```python
from build123d import *

# Parameters (mm, degrees)
F1_DEPTH = 100
F3_DEPTH = 100


with BuildPart() as f1:
    # F0 (on Front) → F1 (new body, symmetric)
    with BuildSketch(Plane.XZ):
        Polygon((450, -325), (450, 325), (150, 325), (150, 75), (-150, 75), (-150, 325), (-450, 325), (-450, -325), align=None)
    extrude(amount=F1_DEPTH, both=True)

    # F2 (on face) → F3 (join, symmetric)
    with BuildSketch(Plane.XZ.offset(100)):
        Polygon((-450, 325), (-450, -325), (-150, -325), align=None)
        Polygon((450, 325), (150, -325), (450, -325), align=None)
    extrude(amount=F3_DEPTH, both=True)


solid = f1.part
```
Could you check a few things on this model? Use its own coordinates, in mm. A direction names the side the tool comes from. Give positions to 0.01 mm unless a question says otherwise; leave off trailing zeros. Order: outer loops, then holes, each group sorted by start corner. A loop starts at its lowest first (then second) coordinate and runs counter-clockwise, first axis right, second up.
Q1. If I drill on line 1 along X through (y, z) = (28, 139); line 2 along Y through (x, z) = (222, 250.5); line 3 along Z through (x, y) = (-42.5, -1.5), over which ranges is the centre line in solid material (lowest first)?
Q2. Suppose I cut it at B-B, the plane z = 149. Write out the boundary of the cut face in (x, y).
Q3. I'm going to push a flat-ended pin straight in: P1, Ø10, axis at x = -122, z = -181.5, coming from the -Y side. Where does the tip first touch, or does it pass through?
Q4. Suppose I cut it at C-C, the plane y = -23.5. Write out the boundary of the cut face in (x, z), and give its area (3 significant figures).
Q5. Suppose I cut it at D-D, the plane z = -255. Write out the boundary of the cut face in (x, y).
Q6. We'd pull the mould along X, two halves only. Please class faces 4 (the flat face through (450, -52, -5)), 5 (the flat face through (-6, -52, -325)), 6 (the flat face through (-297.9, -149.3, -4.55)), 7 (the flat face through (-150, -1, 198)): +X half, -X half, draft (parallel to the pull), parting line (faces both ways), or undercut.
Q7. For faces 1 (the flat face through (-6, -100, 5)), 2 (the flat face through (365, -200, -140)), 3 (the flat face through (150, -1, 202)), which set-ups out of +Z, -Z, +X, -X, +Y, -Y let a thin tool reach every point of the face, with its end or its side?
Q8. Suppose I cut it at A-A, the plane y = -173. Write out the boundary of the cut face in (x, z), and give its area (3 significant figures).
Solution:
1. line 1: x = -450 to -150, 150 to 450
1. line 2: y = -100 to 100
1. line 3: z = -325 to 75
2. outline: (-450, -200) - (-368.77, -200) - (-368.77, -100) - (-150, -100) - (-150, 100) - (-450, 100) - close; (150, -100) - (368.77, -100) - (368.77, -200) - (450, -200) - (450, 100) - (150, 100) - close
3. P1: stops at y = -100
4. outline: (-450, -325) - (450, -325) - (450, 325) - (150, 325) - (150, 75) - (-150, 75) - (-150, 325) - (-450, 325) - close
4. area: 510,000 mm2
5. outline: (-450, -200) - (-182.31, -200) - (-182.31, -100) - (182.31, -100) - (182.31, -200) - (450, -200) - (450, 100) - (-450, 100) - close
6. face 4: +X half
6. face 5: draft
6. face 6: undercut
6. face 7: undercut
7. face 1: +Z, -Y
7. face 2: +Z, -Z, +X, -X, -Y
7. face 3: +Z, +Y, -Y
8. outline: (-450, -325) - (-150, -325) - (-450, 325) - close; (150, -325) - (450, -325) - (450, 325) - close
8. area: 195,000 mm2
